Autodesk Inventor part; units mm, degrees
ref_plane "Work Plane1" through (0, 0, -9) normal (0, 0, 1) x (1, 0, 0)
ref_plane "YZ Plane" through (0, 0, 0) normal (1, 0, 0) x (0, 1, 0)
ref_plane "XZ Plane" through (0, 0, 0) normal (0, 1, 0) x (-1, 0, 0)
sketch "Sketch1" plane through (0, 0, 0) normal (0, 0, 1) x (1, 0, 0)
  line L0 (-10, -20) -> (10, -20)
  line L1 (10, -20) -> (10, 20)
  line L2 (10, 20) -> (-10, 20)
  line L3 (-10, 20) -> (-10, -20)
  line L4 (-10, -20) -> (10, 20) construction
  line L5 (10, -20) -> (-10, 20) construction
  point P0 (0, 0)
  dimension "d0" = 40
  dimension "d1" = 20
extrude "Extrusion1" add sketch "Sketch1" against normal blind 38
fillet "Fillet2" radius 1 4 edges at (-10, 20, -19) (10, 20, -19) (-10, -20, -19) (10, -20, -19)
ref_plane "Work Plane1" through (0, 0, -9) normal (0, 0, 1) x (1, 0, 0)
sketch "Sketch2" plane through (0, 0, -9) normal (0, 0, 1) x (1, 0, 0)
  line L0 (10, -19) -> (-10, -19)
  line L1 (-10, -19) -> (-10, -27.5)
  line L2 (-10, -27.5) -> (10, -27.5)
  line L3 (10, -27.5) -> (10, -19)
  line L4 (-10, 19) -> (-10, -19)
  line L5 (-9, -20) -> (9, -20)
  line L6 (10, 19) -> (10, -19)
  line L7 (10, 0) -> (-10, 0)
  line L8 (10, 19) -> (-10, 19)
  line L9 (-10, 19) -> (-10, 27.5)
  line L10 (-10, 27.5) -> (10, 27.5)
  line L11 (10, 27.5) -> (10, 19)
  line L12 (10, -23) -> (-10, -23) construction
  line L13 (0, -27.5) -> (0, -20) construction
  circle A0 centre (5.5, -23) radius 2.5
  line L14 (8, -20.5) -> (3, -20.5) construction
  line L15 (3, -20.5) -> (3, -25.5) construction
  line L16 (3, -25.5) -> (8, -25.5) construction
  line L17 (8, -25.5) -> (8, -20.5) construction
  line L18 (8, -20.5) -> (3, -25.5) construction
  line L19 (3, -20.5) -> (8, -25.5) construction
  line L20 (7.25, -27.5) -> (3.75, -27.5)
  line L21 (3.75, -27.5) -> (3.75, -24.7854)
  line L22 (3.75, -24.7854) -> (7.25, -24.7854)
  line L23 (7.25, -24.7854) -> (7.25, -27.5)
  line L24 (5.5, -24.7854) -> (5.5, -23) construction
  circle A1 centre (-5.5, -23) radius 2.5
  line L25 (-3.75, -27.5) -> (-3.75, -24.7854)
  line L26 (-7.25, -24.7854) -> (-7.25, -27.5)
  circle A2 centre (5.5, 23) radius 2.5
  line L27 (3.75, 27.5) -> (3.75, 24.7854)
  line L28 (7.25, 24.7854) -> (7.25, 27.5)
  line L29 (-7.25, 24.7854) -> (-7.25, 27.5)
  line L30 (-3.75, 27.5) -> (-3.75, 24.7854)
  circle A3 centre (-5.5, 23) radius 2.5
  point P0 (0, 0)
  dimension "d8" = 5
  dimension "d7" = 7.5
  dimension "d9" = 2
  dimension "d10" = 2
  dimension "d11" = 3.5
extrude "Extrusion2" add sketch "Sketch2" against normal blind 2.5 contours L3 L2 L23 A0 L21 L25 A1 L26 L1 L0 | L8 L9 L10 L29 A3 L30 L27 A2 L28 L11
fillet "Fillet3" radius 1.5 4 edges at (-10, 27.5, -10.25) (10, 27.5, -10.25) (-10, -27.5, -10.25) (10, -27.5, -10.25)
sketch "Sketch3" plane through (0, 0, -38) normal (0, 0, -1) x (-1, 0, 0)
  arc A0 (-10, -19) -> (-9, -20) centre (-9, -19) ccw
  line L0 (-9, -20) -> (9, -20)
  arc A1 (9, -20) -> (10, -19) centre (9, -19) ccw
  line L1 (10, -19) -> (10, 19)
  arc A2 (10, 19) -> (9, 20) centre (9, 19) ccw
  line L2 (9, 20) -> (-9, 20)
  arc A3 (-9, 20) -> (-10, 19) centre (-9, 19) ccw
  line L3 (-10, 19) -> (-10, -19)
  circle A4 centre (9, 19) radius 1.5
  circle A5 centre (-9, 19) radius 1.5
  circle A6 centre (9, -19) radius 1.5
  circle A7 centre (-9, -19) radius 1.5
  point P0 (0, 0)
  dimension "d15" = 3
extrude "Extrusion3" cut sketch "Sketch3" against normal blind 1 contours L3 A7 L0 A0 | A0 L0 A7 L3 | A5 L2 A3 L3 | L3 A3 L2 A5 | A6 L1 A1 L0 | L0 A1 L1 A6 | A4 L1 A2 L2 | L2 A2 L1 A4
sketch "Sketch4" plane through (10, -19, 0) normal (1, 0, 0) x (0, 0, -1)
  line L0 (9, 0) -> (9, -7)
  line L1 (9, 39) -> (9, 38)
  line L2 (9, 0) -> (9, 38) construction
  line L3 (9, -1) -> (0, -1)
  line L4 (4.5, -1) -> (0, 3.5)
  line L5 (0, 0) -> (0, 38)
  line L6 (0, -1) -> (0, 0)
  point P0 (0, 19)
  dimension "d18" = 4.5
  dimension "d19" = 4.5
extrude "Extrusion4" cut sketch "Sketch4" against normal through all
sketch "Sketch5" plane through (0, 0, 0) normal (0, 0, 1) x (1, 0, 0)
  circle A0 centre (0, 10) radius 7.9
  line L0 (10, -15.5) -> (10, 19)
  line L1 (-10, 19) -> (-10, -15.5)
  line L2 (9, 20) -> (-9, 20)
  line L3 (0, 17.9) -> (0, -5.6)
  circle A1 centre (0, -5.6) radius 4
  line L4 (7.6491, 8.025) -> (3.873, -6.6)
  line L5 (-7.6491, 8.025) -> (-3.873, -6.6)
  point P0 (0, 0)
  dimension "d22" = 15.8
  dimension "d23" = 10
  dimension "d24" = 10
  dimension "d25" = 10
  dimension "d26" = 23.5
  dimension "d27" = 8
extrude "Extrusion5" add sketch "Sketch5" along normal blind 0.5
sketch "Sketch6" plane through (0, 0, 0.5) normal (0, 0, 1) x (1, 0, 0)
  arc A0 (7.6491, 8.025) -> (-7.6491, 8.025) centre (0, 10) ccw
  circle A1 centre (0, 10) radius 6.17
  point P0 (0, 0)
  dimension "d30" = 12.34
extrude "Extrusion6" add sketch "Sketch6" along normal blind 1 draft -50
sketch "Sketch7" plane through (0, 10, 1.5) normal (0, 0, 1) x (1, 0, 0)
  circle A0 centre (0, 0) radius 4.9782
  circle A1 centre (0, 0) radius 3
  point P0 (0, -10)
  dimension "d33" = 6
extrude "Extrusion7" add sketch "Sketch7" along normal blind 4 contours A1
sketch "Sketch8" plane through (0, 0, 0) normal (1, 0, 0) x (0, 1, 0)
  line L0 (-24.7854, -9) -> (-27.5, -9)
  line L1 (-27, -9) -> (-20, -6)
  line L2 (-20, -9) -> (-20, -4.5)
  line L3 (-20, -9) -> (-20, -6)
  line L4 (-20, -9) -> (-27, -9)
  point P0 (0, 0)
  dimension "d36" = 3
  dimension "d37" = 7
extrude "Extrusion8" add sketch "Sketch8" along normal mid plane 1.4
mirror "Mirror1" about plane through (0, 0, 0) normal (0, 1, 0) of "Extrusion8"
sketch "Sketch9" plane through (-9, 20, -11.5) normal (0, 1, 0) x (1, 0, 0)
  line L0 (5.25, 0) -> (12.75, 0)
  line L1 (9, 0) -> (9, 26.5) construction
  line L2 (1.118, 26.5) -> (16.882, 26.5)
  line L3 (12.5, 19.7) -> (5.5, 19.7)
  line L4 (5.5, 19.7) -> (5.5, 24)
  line L5 (5.5, 24) -> (12.5, 24)
  line L6 (12.5, 24) -> (12.5, 19.7)
  line L7 (12.5, 19.7) -> (5.5, 24) construction
  line L8 (5.5, 19.7) -> (12.5, 24) construction
  point P0 (9, -11.5)
  point P1 (9, 21.85)
  dimension "d40" = 2.5
  dimension "d41" = 7
  dimension "d42" = 4.3
extrude "Extrusion9" add sketch "Sketch9" along normal blind 7 draft -5
fillet "Fillet4" radius 1 4 edges at (3.1938, 23.5, -31.5062) (3.1938, 23.5, -35.1938) (-3.1938, 23.5, -31.5062) (-3.1938, 23.5, -35.1938)
chamfer "Chamfer1" distance 1 angle 45 5 edges at (0, 20, 0) (-9.7071, 19.7071, 0) (-10, 1.75, 0) (9.7071, 19.7071, 0) (10, 1.75, 0)
equation "\"d10\" = d9"
equation "\"d19\" = d18"
equation "\"d24\" = d23"
equation "\"d25\" = d23"
properties part number "DatanS1213AnalogFeedback"
Verification items for the finished model (mm, model axes). A direction names the side the tool comes from. Coordinates: 2 decimals unless noted, no trailing zeros. Order: outer loops, then holes, each group sorted by start corner. A loop starts at its lowest first (then second) coordinate and runs counter-clockwise, first axis right, second up.
Item 1: Depth check by flat-ended pin: pin 1 (12 mm diameter, centred on x = 3, y = -19.5, fed in from +Z); pin 2 (5 mm diameter, centred on x = -6.5, z = -25, fed in from -Y); pin 3 (8 mm diameter, centred on x = 5.5, y = -23, fed in from +Z). Enter the tip coordinate at first touch or a pass-through.
Filled in:
pin 1: stops at z = 0
pin 2: stops at y = -20
pin 3: stops at z = -3.5
Item 2: Section check C-C, the plane y = 10. Enter the section's corners in (x, z), then the cut area to 3 significant figures.
Filled in:
outline: (-10, -38) - (10, -38) - (10, -1) - (9, 0) - (7.9, 0) - (7.9, 0.5) - (6.17, 0.5) - (4.98, 1.5) - (3, 1.5) - (3, 5.5) - (-3, 5.5) - (-3, 1.5) - (-4.98, 1.5) - (-6.17, 0.5) - (-7.9, 0.5) - (-7.9, 0) - (-9, 0) - (-10, -1) - close
area: 802 mm2
Item 3: Access from +Z, -Z, +X, -X, +Y, -Y to the whole of each face (thin tool, end or side, straight path). Record for faces 1 (the face through (-3.75, -26, -10)), 2 (the face through (0, 27, -33)), 3 (the face through (-6, -2, 0)), 4 (the face through (0, 20, -5)).
Filled in:
face 1: +Z, -Z, -Y
face 2: -Z, +X, -X, +Y
face 3: +Z
face 4: +Z, +Y
Item 4: Release check for a two-part mould opening along X. For faces 5 (the face through (-3.266, 22.673, -33.334)), 6 (the face through (-0.202, 17.897, 0.246)), 7 (the face through (7.25, 26, -10)), 8 (the face through (0, 0, -38)) record: +X half, -X half, draft (parallel to the pull), parting line (faces both ways), or undercut.
Filled in:
face 5: -X half
face 6: parting line
face 7: undercut
face 8: draft
Item 5: Section check A-A, the plane z = -20.5. Enter the section's corners in (x, y), then the cut area to 3 significant figures.
Filled in:
outline: (-10, -19) arc R1 ccw to (-9, -20) - (9, -20) arc R1 ccw to (10, -19) - (10, 19) arc R1 ccw to (9, 20) - (-9, 20) arc R1 ccw to (-10, 19) - close
area: 799 mm2
Item 6: Section check D-D, the plane y = 23. Give the number of separate pieces and of enclosed holes in the cut face, then the cut area to 3 significant figures.
Filled in:
separate pieces: 4
enclosed holes: 0
area: 51.0 mm2
Item 7: Section check B-B, the plane y = -23. Enter the section's corners in (x, z), then the cut area to 3 significant figures.
Filled in:
outline: (-10, -11.5) - (-8, -11.5) - (-8, -9) - (-10, -9) - close; (-3, -11.5) - (3, -11.5) - (3, -9) - (0.7, -9) - (0.7, -7.29) - (-0.7, -7.29) - (-0.7, -9) - (-3, -9) - close; (8, -11.5) - (10, -11.5) - (10, -9) - (8, -9) - close
area: 27.4 mm2
Item 8: Material ranges on L1, parallel to X at y = 23, z = -10.25; L2, parallel to Y at x = 3.5, z = -25; L3, parallel to Z at x = 7.5, y = -15.5, recorded low to high.
Filled in:
L1: x = -10 to -8, -3 to 3, 8 to 10
L2: y = -20 to 20
L3: z = -38 to 0
